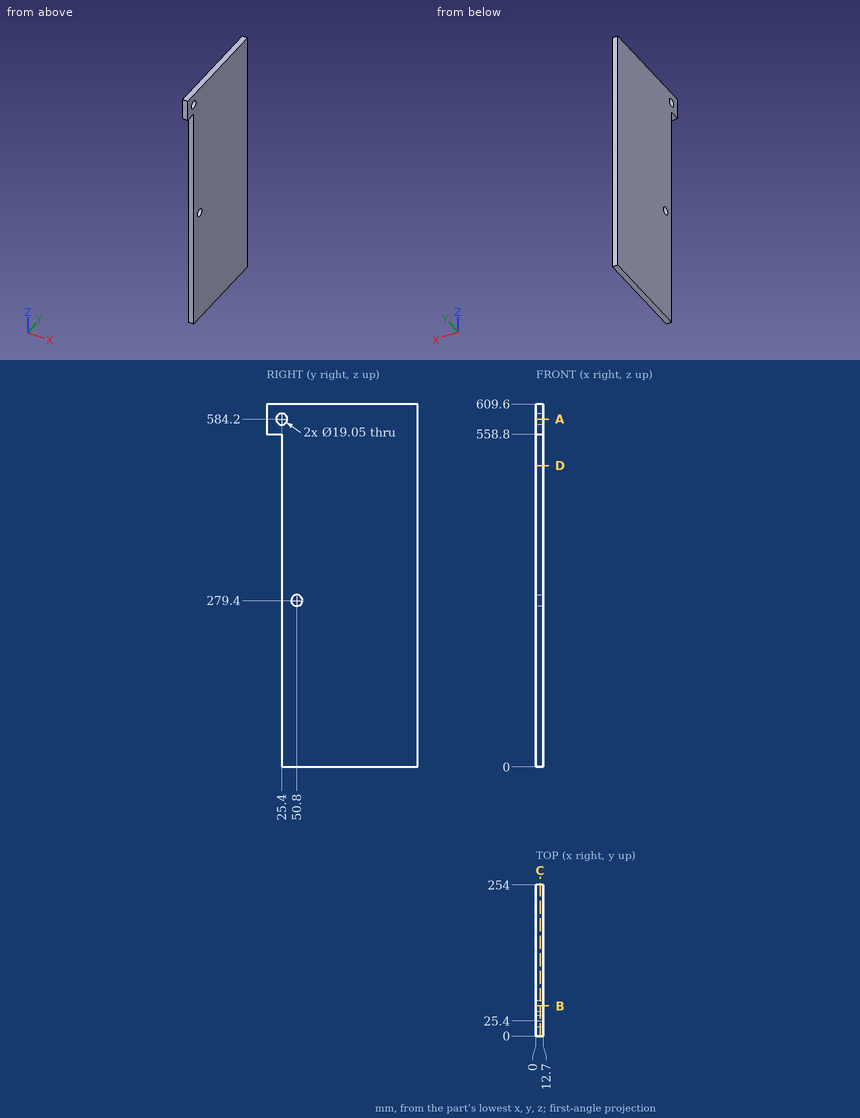
For this review, use the dimensioned drawing (mm, ordinates from the lowest corner) and the shaded views. Round coordinates to 2 decimals unless told otherwise and drop trailing zeros. Loops run counter-clockwise (first coordinate to the right, second up) from the corner with the lowest first, then second, coordinate; pieces in that order, holes last. Notation, with made-up numbers: (2.25, 61) -> (47.25, 61) arc R29 ccw to (47.25, 86) -> close; hole circle Ø2 at (88.5, 46.25). An arc over 180 degrees is marked (long way). Write item = value, one per line. Start each with the question number.
Item 1: Take a section at A-A on z = 584.2. Give the boundary of the cut face in (x, y) (3 decimals).
Item 2: Insertion check: pin 1 (4 mm diameter, centred on x = 4, z = 383, fed in from -Y); pin 2 (17 mm diameter, centred on y = 50.8, z = 279.4, fed in from +X); pin 3 (25 mm diameter, centred on y = 25.4, z = 584.2, fed in from -X); pin 4 (4 mm diameter, centred on x = 5.5, y = 10, fed in from -Z). Each pin has a flat end and moves straight along its axis. Give the tip position at first contact, or say it passes through.
Item 3: Take a section at B-B on y = 50.8. Give the boundary of the cut face in (x, z) (3 decimals), plus the area to 3 significant figures.
Item 4: Take a section at D-D on z = 506. Give the boundary of the cut face in (x, y), plus the area to 3 significant figures.
Item 5: To check wall thickness, follow L1, parallel to Y at x = 11.75, z = 280.5; L2, parallel to Y at x = 4.5, z = 584.2 (3 decimals); L3, parallel to Y at x = 1.75, z = 52. State the ranges of each line that lie inside material, in increasing order.
Item 6: Take a section at C-C on x = 7.25. Give the boundary of the cut face in (y, z) (3 decimals).
Result:
q1.outline = (0, 0) -> (12.7, 0) -> (12.7, 15.875) -> (0, 15.875) -> close; (0, 34.925) -> (12.7, 34.925) -> (12.7, 254) -> (0, 254) -> close
q2.pin_1 = 25.4
q2.pin_2 = through
q2.pin_3 = 0
q2.pin_4 = 558.8
q3.outline = (0, 0) -> (12.7, 0) -> (12.7, 269.875) -> (0, 269.875) -> close; (0, 288.925) -> (12.7, 288.925) -> (12.7, 609.6) -> (0, 609.6) -> close
q3.area = 7,500 mm²
q4.outline = (0, 25.4) -> (12.7, 25.4) -> (12.7, 254) -> (0, 254) -> close
q4.area = 2,900 mm²
q5.L1 = 25.4 to 41.34, 60.26 to 254
q5.L2 = 0 to 15.875, 34.925 to 254
q5.L3 = 25.4 to 254
q6.outline = (0, 558.8) -> (25.4, 558.8) -> (25.4, 0) -> (254, 0) -> (254, 609.6) -> (0, 609.6) -> close; hole circle Ø19.05 at (25.4, 584.2); hole circle Ø19.05 at (50.8, 279.4)
